```python
from build123d import *

# Parameters (mm, degrees)
SKETCH_1_R                   = 60
EXTRUDE_1_DEPTH              = 8
EXTRUDE_START                = -8
EXTRUDE_2_DEPTH              = 8
FILLET_1_R                   = 2
HOLE_WIZARD_M3_1_D           = 3.4
HOLE_WIZARD_M3_1_CSINK_D     = 3.45
HOLE_WIZARD_M3_1_CSINK_ANGLE = 82
SKETCH_8_R                   = 10.5
CUT_EXTRUDE_1_DEPTH          = 89.820042783


with BuildPart() as part:
    # ｽｹｯﾁ1 → ﾎﾞｽ - 押し出し1 (new body)
    with BuildSketch(Plane.XY):
        Circle(SKETCH_1_R)
    extrude(amount=EXTRUDE_1_DEPTH)

    # ｽｹｯﾁ2 → ﾎﾞｽ - 押し出し2 (add)
    with BuildSketch(Plane.XY.offset(8).offset(EXTRUDE_START)):
        with BuildLine():
            Line((10.41889066, 59.088465181), (11.287131548, 64.012503946))
            ThreePointArc((11.287131548, 64.012503946), (0, 65), (-11.287131548, 64.012503946))
            Line((-11.287131548, 64.012503946), (-10.41889066, 59.088465181))
            ThreePointArc((-10.41889066, 59.088465181), (0, 60), (10.41889066, 59.088465181))
        make_face()
        with BuildLine():
            Line((10.41889066, -59.088465181), (11.287131548, -64.012503946))
            ThreePointArc((11.287131548, -64.012503946), (0, -65), (-11.287131548, -64.012503946))
            Line((-11.287131548, -64.012503946), (-10.41889066, -59.088465181))
            ThreePointArc((-10.41889066, -59.088465181), (0, -60), (10.41889066, -59.088465181))
        make_face()
    extrude(amount=EXTRUDE_2_DEPTH)

    # ﾌｨﾚｯﾄ1
    fillet_1_edges = [part.edges().sort_by_distance(p)[0] for p in [
        (-10.41889066, -59.088465181, 4),
        (10.41889066, -59.088465181, 4),
        (11.287131548, -64.012503946, 4),
        (-11.287131548, -64.012503946, 4),
        (10.41889066, 59.088465181, 4),
        (-10.41889066, 59.088465181, 4),
        (-11.287131548, 64.012503946, 4),
        (11.287131548, 64.012503946, 4),
    ]]
    fillet(fillet_1_edges, radius=FILLET_1_R)

    # M3 すきま穴1 (through all)
    with Locations(Plane(origin=(0, 0, 0), x_dir=(-1, 0, 0), z_dir=(0, 0, -1))):
        with Locations((0, 54), (46.765371804, 27), (46.765371804, -27), (0, -54), (-46.765371804, -27), (-46.765371804, 27)):
            CounterSinkHole(HOLE_WIZARD_M3_1_D / 2, HOLE_WIZARD_M3_1_CSINK_D / 2, counter_sink_angle=HOLE_WIZARD_M3_1_CSINK_ANGLE)

    # ｽｹｯﾁ8 → ｶｯﾄ - 押し出し1 (cut, through all)
    with BuildSketch(Plane(origin=(0, 0, 0), x_dir=(-1, 0, 0), z_dir=(0, 0, -1))):
        with Locations((0, 28)):
            Circle(SKETCH_8_R)
        with Locations((24.248711306, -14)):
            Circle(SKETCH_8_R)
        with Locations((-24.248711306, -14)):
            Circle(SKETCH_8_R)
    extrude(amount=-CUT_EXTRUDE_1_DEPTH, mode=Mode.SUBTRACT)


solid = part.part
```
Verification items for the finished model (mm, model axes). Round coordinates to 2 decimals unless told otherwise and drop trailing zeros. Write each loop counter-clockwise with the first axis right and the second up, starting at its lowest first coordinate (ties: lowest second). Pieces come first, ordered by that corner, then holes.
1. Gauge pin test, flat ends, axial feed: P1, Ø1.5, axis at x = -8.5, z = 1.5, coming from the +Y side; P2, Ø3, axis at y = -17.5, z = 5.5, coming from the +X side; P3, Ø3, axis at y = 24, z = 1, coming from the +X side. Record the tip position at first contact, or that the pin passes through.
2. Scan lines: L1, parallel to Y at x = 1.5, z = 2; L2, parallel to Y at x = 46, z = 5.25; L3, parallel to X at y = -27, z = 6.25. Record each from-to range of solid material in increasing order.
3. Section check B-B on z = 5.5. State how many separate pieces and enclosed holes the cut face has, plus the area to 3 significant figures.
4. Section check A-A on x = 0. Enter the section's corners in (y, z) (3 decimals).
5. Draft check along Y on faces 1 (the cylindrical face through (-21.97, -24.25, 3.94)), 2 (the cylindrical face through (0, -65, 4)), 3 (the cylindrical face through (59.99, -1.15, 3.94)), 4 (the flat face through (-1, 1, 0)). Enter one of: +Y half, -Y half, draft (parallel to the pull), parting line (faces both ways), or undercut.
6. Section check D-D on y = -54. Enter the section's corners in (x, z) (3 decimals).
7. Section check C-C on y = -23. Enter the section's corners in (x, z), plus the area to 3 significant figures.
Answer:
1. P1: stops at y = 64.54
1. P2: stops at x = 57.83
1. P3: stops at x = 55.62
2. L1: y = -64.98 to -54.8, -53.2 to 17.61, 38.39 to 53.2, 54.8 to 64.98
2. L2: y = -38.52 to -28.52, -25.48 to 25.48, 28.52 to 38.52
2. L3: x = -53.58 to -48.47, -45.07 to 45.07, 48.47 to 53.58
3. separate pieces: 1
3. enclosed holes: 9
3. area: 10,400 mm2
4. outline: (-65, 0) - (-55.725, 0) - (-55.7, 0.029) - (-55.7, 8) - (-65, 8) - close; (-52.3, 0.029) - (-52.275, 0) - (17.5, 0) - (17.5, 8) - (-52.3, 8) - close; (38.5, 0) - (52.275, 0) - (52.3, 0.029) - (52.3, 8) - (38.5, 8) - close; (55.7, 0.029) - (55.725, 0) - (65, 0) - (65, 8) - (55.7, 8) - close
5. face 1: undercut
5. face 2: -Y half
5. face 3: parting line
5. face 4: draft
6. outline: (-26.153, 0) - (-1.725, 0) - (-1.7, 0.029) - (-1.7, 8) - (-26.153, 8) - close; (1.7, 0.029) - (1.725, 0) - (26.153, 0) - (26.153, 8) - (1.7, 8) - close
7. outline: (-55.42, 0) - (-29.66, 0) - (-29.66, 8) - (-55.42, 8) - close; (-18.84, 0) - (18.84, 0) - (18.84, 8) - (-18.84, 8) - close; (29.66, 0) - (55.42, 0) - (55.42, 8) - (29.66, 8) - close
7. area: 714 mm2
